from build123d import *

# Parameters (mm, degrees)
CROQUIS2_R              = 65
SALIENTE_EXTRUIR1_DEPTH = 4
CORTAR_EXTRUIR6_REACH   = 94.011
CROQUIS3_W              = 4
CROQUIS3_H              = 10.2
CROQUIS4_R              = 2
CORTAR_EXTRUIR7_DEPTH   = 10


with BuildPart() as part:
    # Croquis2 → Saliente-Extruir1 (new body)
    with BuildSketch(Plane(origin=(0, 0, 0), x_dir=(1, 0, 0), z_dir=(0, 1, 0))):
        with Locations(Location((0, 0, 0), (0, 0, 270))):
            Circle(CROQUIS2_R)
    extrude(amount=SALIENTE_EXTRUIR1_DEPTH)

    # Croquis3 → Cortar-Extruir6 (cut, up to next)
    with BuildSketch(Plane(origin=(0, 4, 0), x_dir=(1, 0, 0), z_dir=(0, 1, 0)), mode=Mode.PRIVATE) as cortar_extruir6_sk1:
        with Locations((-37, 12.5)):
            Rectangle(CROQUIS3_W, CROQUIS3_H)
    cortar_extruir6_tool1 = extrude(cortar_extruir6_sk1.sketch, amount=-CORTAR_EXTRUIR6_REACH, mode=Mode.PRIVATE) & part.part
    # Croquis3 → Cortar-Extruir6 (cut, up to next)
    with BuildSketch(Plane(origin=(0, 4, 0), x_dir=(1, 0, 0), z_dir=(0, 1, 0)), mode=Mode.PRIVATE) as cortar_extruir6_sk2:
        with Locations((-37, -12.7)):
            Rectangle(CROQUIS3_W, CROQUIS3_H)
    cortar_extruir6_tool2 = extrude(cortar_extruir6_sk2.sketch, amount=-CORTAR_EXTRUIR6_REACH, mode=Mode.PRIVATE) & part.part
    # Croquis3 → Cortar-Extruir6 (cut, up to next)
    with BuildSketch(Plane(origin=(0, 4, 0), x_dir=(1, 0, 0), z_dir=(0, 1, 0)), mode=Mode.PRIVATE) as cortar_extruir6_sk3:
        with Locations((-37, -37.9)):
            Rectangle(CROQUIS3_W, CROQUIS3_H)
    cortar_extruir6_tool3 = extrude(cortar_extruir6_sk3.sketch, amount=-CORTAR_EXTRUIR6_REACH, mode=Mode.PRIVATE) & part.part
    # Croquis3 → Cortar-Extruir6 (cut, up to next)
    with BuildSketch(Plane(origin=(0, 4, 0), x_dir=(1, 0, 0), z_dir=(0, 1, 0)), mode=Mode.PRIVATE) as cortar_extruir6_sk4:
        with Locations((-37, 37.7)):
            Rectangle(CROQUIS3_W, CROQUIS3_H)
    cortar_extruir6_tool4 = extrude(cortar_extruir6_sk4.sketch, amount=-CORTAR_EXTRUIR6_REACH, mode=Mode.PRIVATE) & part.part
    # Croquis3 → Cortar-Extruir6 (cut, up to next)
    with BuildSketch(Plane(origin=(0, 4, 0), x_dir=(1, 0, 0), z_dir=(0, 1, 0)), mode=Mode.PRIVATE) as cortar_extruir6_sk5:
        with Locations((37, 37.7)):
            Rectangle(CROQUIS3_W, CROQUIS3_H)
    cortar_extruir6_tool5 = extrude(cortar_extruir6_sk5.sketch, amount=-CORTAR_EXTRUIR6_REACH, mode=Mode.PRIVATE) & part.part
    # Croquis3 → Cortar-Extruir6 (cut, up to next)
    with BuildSketch(Plane(origin=(0, 4, 0), x_dir=(1, 0, 0), z_dir=(0, 1, 0)), mode=Mode.PRIVATE) as cortar_extruir6_sk6:
        with Locations((37, 12.5)):
            Rectangle(CROQUIS3_W, CROQUIS3_H)
    cortar_extruir6_tool6 = extrude(cortar_extruir6_sk6.sketch, amount=-CORTAR_EXTRUIR6_REACH, mode=Mode.PRIVATE) & part.part
    # Croquis3 → Cortar-Extruir6 (cut, up to next)
    with BuildSketch(Plane(origin=(0, 4, 0), x_dir=(1, 0, 0), z_dir=(0, 1, 0)), mode=Mode.PRIVATE) as cortar_extruir6_sk7:
        with Locations((37, -12.7)):
            Rectangle(CROQUIS3_W, CROQUIS3_H)
    cortar_extruir6_tool7 = extrude(cortar_extruir6_sk7.sketch, amount=-CORTAR_EXTRUIR6_REACH, mode=Mode.PRIVATE) & part.part
    # Croquis3 → Cortar-Extruir6 (cut, up to next)
    with BuildSketch(Plane(origin=(0, 4, 0), x_dir=(1, 0, 0), z_dir=(0, 1, 0)), mode=Mode.PRIVATE) as cortar_extruir6_sk8:
        with Locations((37, -37.9)):
            Rectangle(CROQUIS3_W, CROQUIS3_H)
    cortar_extruir6_tool8 = extrude(cortar_extruir6_sk8.sketch, amount=-CORTAR_EXTRUIR6_REACH, mode=Mode.PRIVATE) & part.part
    add(cortar_extruir6_tool1.solids().sort_by_distance((-37, 4, -12.5))[0], mode=Mode.SUBTRACT)
    add(cortar_extruir6_tool2.solids().sort_by_distance((-37, 4, 12.7))[0], mode=Mode.SUBTRACT)
    add(cortar_extruir6_tool3.solids().sort_by_distance((-37, 4, 37.9))[0], mode=Mode.SUBTRACT)
    add(cortar_extruir6_tool4.solids().sort_by_distance((-37, 4, -37.7))[0], mode=Mode.SUBTRACT)
    add(cortar_extruir6_tool5.solids().sort_by_distance((37, 4, -37.7))[0], mode=Mode.SUBTRACT)
    add(cortar_extruir6_tool6.solids().sort_by_distance((37, 4, -12.5))[0], mode=Mode.SUBTRACT)
    add(cortar_extruir6_tool7.solids().sort_by_distance((37, 4, 12.7))[0], mode=Mode.SUBTRACT)
    add(cortar_extruir6_tool8.solids().sort_by_distance((37, 4, 37.9))[0], mode=Mode.SUBTRACT)

    # Croquis4 → Cortar-Extruir7 (cut)
    with BuildSketch(Plane(origin=(0, 4, 0), x_dir=(1, 0, 0), z_dir=(0, 1, 0))):
        with Locations(Location((0, 0, 0), (0, 0, 270))):
            Circle(CROQUIS4_R)
    extrude(amount=-CORTAR_EXTRUIR7_DEPTH, mode=Mode.SUBTRACT)


solid = part.part
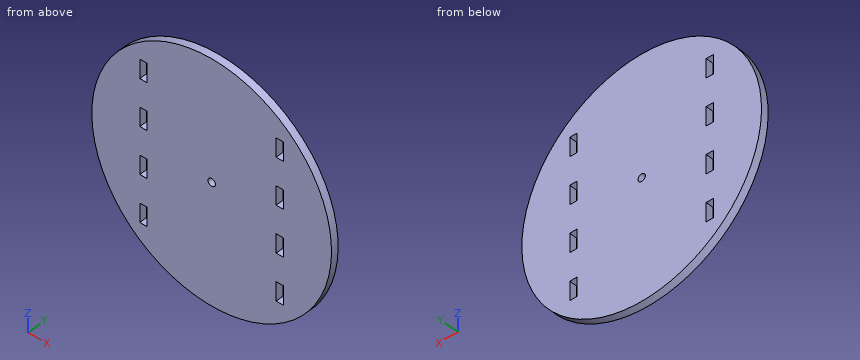
Input: part model. Units: mm. Frame: model coordinates. Coordinates: 2 decimals unless noted, no trailing zeros. Loops run counter-clockwise (first coordinate to the right, second up) from the corner with the lowest first, then second, coordinate; pieces in that order, holes last.
Q1. Cut plane A-A (y = 2.65). Give the number of separate pieces and of enclosed holes in the cut face, then the cut area to 3 significant figures.
Q2. Cut plane D-D (x = -18). Output: boundary loops of the cut face in (y, z), then the cut area to 3 significant figures.
Q3. Material intervals for line 1 (Z direction, x = -38, y = 0.85); line 2 (X direction, y = 0.5, z = 33.5); line 3 (X direction, y = 2.2, z = 0), sorted ascending.
Q4. Contact query for flat-ended pins moving along their axis: pin 1 (1.2 mm diameter, centred on y = 1.5, z = 10.5, fed in from -X); pin 2 (2 mm diameter, centred on x = -36.5, y = 2, fed in from +Z); pin 3 (2 mm diameter, centred on y = 1, z = -13, fed in from +X). Output: stop coordinate, or through.
Q5. Cut plane B-B (x = 0). Output: boundary loops of the cut face in (y, z).
Q6. Cut plane C-C (z = 0). Output: boundary loops of the cut face in (x, y), then the cut area to 3 significant figures.
Working result:
1. separate pieces: 1
1. enclosed holes: 9
1. area: 12,900 mm2
2. outline: (0, -62.46) - (4, -62.46) - (4, 62.46) - (0, 62.46) - close
2. area: 500 mm2
3. line 1: z = -52.74 to -42.8, -32.6 to -17.6, -7.4 to 7.6, 17.8 to 32.8, 43 to 52.74
3. line 2: x = -55.7 to -39, -35 to 35, 39 to 55.7
3. line 3: x = -65 to -2, 2 to 65
4. pin 1: stops at x = -64.24
4. pin 2: stops at z = 54.45
4. pin 3: stops at x = 63.88
5. outline: (0, -65) - (4, -65) - (4, -2) - (0, -2) - close; (0, 2) - (4, 2) - (4, 65) - (0, 65) - close
6. outline: (-65, 0) - (-2, 0) - (-2, 4) - (-65, 4) - close; (2, 0) - (65, 0) - (65, 4) - (2, 4) - close
6. area: 504 mm2
